from build123d import *

# Parameters (mm, degrees)
F0_W     = 60
F0_H     = 127
F1_DEPTH = 10
F2_R     = 8
F3_R     = 6
F4_DEPTH = 1
F5_W     = 56
F5_H     = 91
F6_DEPTH = 1
F7_W     = 12
F7_H     = 4
F7_R     = 3
F8_DEPTH = 2
F9_R     = 1.99999
F10_R    = 0.5


# Not quite as in the source:
# - a fillet or chamfer is up to 0.001 mm smaller than in the source, because OpenCascade refuses the exact size


with BuildPart() as f1:
    # F0 (on Front) → F1 (new body)
    with BuildSketch(Plane.XZ):
        Rectangle(F0_W, F0_H)
    extrude(amount=F1_DEPTH)

    # F2
    f2_edges = [f1.edges().sort_by_distance(p)[0] for p in [
        (30, -5, 63.5),
        (-30, -5, 63.5),
        (30, -5, -63.5),
        (-30, -5, -63.5),
    ]]
    fillet(f2_edges, radius=F2_R)

    # F3 (on face) → F4 (cut)
    with BuildSketch(Plane.XZ.offset(10)):
        with Locations((0, -52.5)):
            Circle(F3_R)
    extrude(amount=-F4_DEPTH, mode=Mode.SUBTRACT)

    # F5 (on face) → F6 (cut)
    with BuildSketch(Plane.XZ.offset(10)):
        with Locations((0, 1)):
            Rectangle(F5_W, F5_H)
    extrude(amount=-F6_DEPTH, mode=Mode.SUBTRACT)

    # F7 (on face) → F8 (cut)
    with BuildSketch(Plane(origin=(0, 0, -63.5), x_dir=(1, 0, 0), z_dir=(0, 0, -1))):
        with Locations((0, 5)):
            Rectangle(F7_W, F7_H)
        with Locations((16, 5)):
            Rectangle(F7_W, F7_H)
        with Locations((-19, 5)):
            Circle(F7_R)
    extrude(amount=-F8_DEPTH, mode=Mode.SUBTRACT)

    # F9 (radius 2 in the source; OpenCascade refuses exactly that, so slightly less here)
    f9_edges = [f1.edges().sort_by_distance(p)[0] for p in [
        (-6, -7, -62.5),
        (-6, -3, -62.5),
        (6, -7, -62.5),
        (6, -3, -62.5),
    ]]
    fillet(f9_edges, radius=F9_R)

    # F10
    f10_edges = [f1.edges().sort_by_distance(p)[0] for p in [
        (10, -7, -62.5),
        (10, -3, -62.5),
        (22, -3, -62.5),
        (22, -7, -62.5),
    ]]
    fillet(f10_edges, radius=F10_R)


solid = f1.part
Could you check a few things on this model? Use its own coordinates, in mm. A direction names the side the tool comes from. Give positions to 0.01 mm unless a question says otherwise; leave off trailing zeros. Loops run counter-clockwise (first coordinate to the right, second up) from the corner with the lowest first, then second, coordinate; pieces in that order, holes last. Notation, with made-up numbers: M 42,79 L 82,79 A7 ccw 82,88 Z; hole C 72.25,67.25 d7. An arc over 180 degrees is marked long. Answer as a JSON object with one key per item and string values.
Q1. If we mould it in two halves opening along Y, with no side actions, what happens to faces 1 (the flat face through (-19, -5, -61.5)), 2 (the flat face through (-29, -10, 19)), 3 (the cylindrical face through (27.594, -5.07, -61.219))? For each: pulls with the +Y half, pulls with the -Y half, needs draft (parallel to the pull), parting line crosses it, or undercut.
Values found:
{"face 1": "undercut", "face 2": "pulls with the -Y half", "face 3": "needs draft"}
Q2. If I drill on probe 1 along Z at (x, y) = (0, -9.8); probe 2 along Z at (x, y) = (-15, -9.5); probe 3 along Y at (x, z) = (-19, -62.75), over which ranges is the centre line in solid material (lowest first)? Write a range as [from, to].
Values found:
{"probe 1": "z = [-63.5, -58.5], [-46.5, -44.5], [46.5, 63.5]", "probe 2": "z = [-63.5, -44.5], [46.5, 63.5]", "probe 3": "y = [-10, -8], [-2, 0]"}
Q3. Suppose I cut it at B-B, the plane x = 0. List the corners of the cut face in (y, z) for me, plus the area to 3 significant figures.
Values found:
{"outline": "M -10,-63.5 L -7,-63.5 L -7,-61.5 L -3,-61.5 L -3,-63.5 L 0,-63.5 L 0,63.5 L -10,63.5 L -10,46.5 L -9,46.5 L -9,-44.5 L -10,-44.5 L -10,-46.5 L -9,-46.5 L -9,-58.5 L -10,-58.5 Z", "area": "1,160 mm²"}
Q4. For faces 4 (the flat face through (0, -9, -52)), 5 (the flat face through (16, -5, -61.5)), 6 (the cylindrical face through (27.719, -5.07, 61.094)), which set-ups out of +Z, -Z, +X, -X, +Y, -Y let a thin tool reach every point of the face, with its end or its side?
Values found:
{"face 4": "-Y", "face 5": "-Z", "face 6": "+Z, +X, +Y, -Y"}
Q5. Suppose I cut it at D-D, the plane z = -13.5. List the corners of the cut face in (x, y) for me, plus the area to 3 significant figures.
Values found:
{"outline": "M -30,-10 L -28,-10 L -28,-9 L 28,-9 L 28,-10 L 30,-10 L 30,0 L -30,0 Z", "area": "544 mm²"}
Q6. Suppose I cut it at C-C, the plane x = -19. List the corners of the cut face in (y, z) for me.
Values found:
{"outline": "M -10,-63.5 L -8,-63.5 L -8,-61.5 L -2,-61.5 L -2,-63.5 L 0,-63.5 L 0,63.5 L -10,63.5 L -10,46.5 L -9,46.5 L -9,-44.5 L -10,-44.5 Z"}
Q7. For P1, Ø2, axis at x = -1, z = -63, coming from the +Y side; P2, Ø1, axis at y = -5, z = -62, coming from the +X side; P3, Ø3, axis at x = 18.5, y = -5, coming from the -Z side, each with a flat end and sliding along its axis, tell me the tip position at first contact or that it passes through.
Values found:
{"P1": "stops at y = 0", "P2": "stops at x = 27.29", "P3": "stops at z = -61.5"}
Q8. Suppose I cut it at A-A, the plane z = -52.5. List the corners of the cut face in (x, y) for me.
Values found:
{"outline": "M -30,-10 L -6,-10 L -6,-9 L 6,-9 L 6,-10 L 30,-10 L 30,0 L -30,0 Z"}
